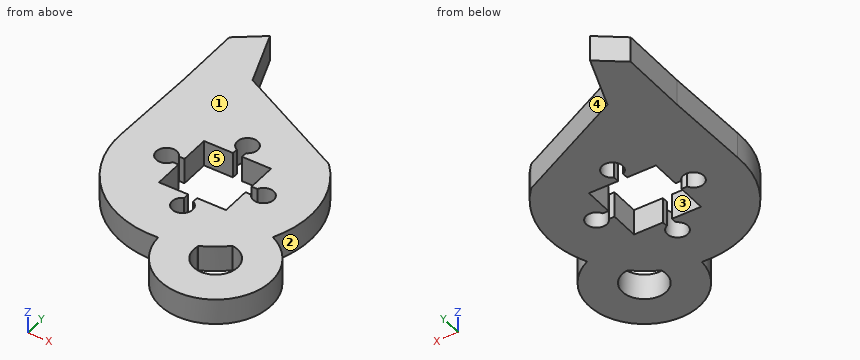
from build123d import *

# Parameters (mm, degrees)
BOSS_EXTRUDE1_DEPTH = 6.35
BOSS_EXTRUDE3_DEPTH = 6.35


with BuildPart() as part:
    # Sketch1 → Boss-Extrude1 (new body)
    with BuildSketch(Plane.XY):
        with BuildLine():
            Line((-23.080739782, 22.623363343), (-23.587362778, 1.111628824))
            ThreePointArc((-23.587362778, 1.111628824), (8.159769108, -22.158916254), (17.23339163, 16.143407769))
            Line((17.23339163, 16.143407769), (-11.238980923, 30.520917168))
            Line((-11.238980923, 30.520917168), (-16.457039411, 44.691234922))
            Line((-16.457039411, 44.691234922), (-23.120633834, 39.693776399))
            Line((-23.120633834, 39.693776399), (-23.080739782, 22.623363343))
        make_face()
        with BuildLine():
            ThreePointArc((1.1176, 9.657085657), (0, 14.478), (-1.1176, 9.657085657))
            Line((-1.1176, 9.657085657), (-1.1176, 8.255))
            Line((-1.1176, 8.255), (-8.255, 8.255))
            Line((-8.255, 8.255), (-8.255, 1.1176))
            Line((-8.255, 1.1176), (-9.657085657, 1.1176))
            ThreePointArc((-9.657085657, 1.1176), (-14.478, 0), (-9.657085657, -1.1176))
            Line((-9.657085657, -1.1176), (-8.255, -1.1176))
            Line((-8.255, -1.1176), (-8.255, -8.255))
            Line((-8.255, -8.255), (-1.1176, -8.255))
            Line((-1.1176, -8.255), (-1.1176, -9.657085657))
            ThreePointArc((-1.1176, -9.657085657), (0, -14.478), (1.1176, -9.657085657))
            Line((1.1176, -9.657085657), (1.1176, -8.255))
            Line((1.1176, -8.255), (8.255, -8.255))
            Line((8.255, -8.255), (8.255, -1.1176))
            Line((8.255, -1.1176), (9.657085657, -1.1176))
            ThreePointArc((9.657085657, -1.1176), (14.478, 0), (9.657085657, 1.1176))
            Line((9.657085657, 1.1176), (8.255, 1.1176))
            Line((8.255, 1.1176), (8.255, 8.255))
            Line((8.255, 8.255), (1.1176, 8.255))
            Line((1.1176, 8.255), (1.1176, 9.657085657))
        make_face(mode=Mode.SUBTRACT)
    extrude(amount=BOSS_EXTRUDE1_DEPTH)

    # Sketch2 → Boss-Extrude3 (add)
    with BuildSketch(Plane(origin=(0, 0, 0), x_dir=(-1, 0, 0), z_dir=(0, 0, -1))):
        with BuildLine():
            ThreePointArc((-13.902877587, -9.175702687), (-24.867617177, -32.651605631), (-1.941453441, -20.57954907))
            ThreePointArc((-1.941453441, -20.57954907), (-6.682478708, -17.156714595), (-10.105313182, -21.897739863))
            ThreePointArc((-10.105313182, -21.897739863), (-19.161295375, -26.666279881), (-14.830152685, -17.393147165))
            ThreePointArc((-14.830152685, -17.393147165), (-10.257792897, -13.748062475), (-13.902877587, -9.175702687))
        make_face()
    extrude(amount=-BOSS_EXTRUDE3_DEPTH)


solid = part.part
The model under review builds one solid part; all positions refer to its coordinate system, in mm. Face numbers are marked on the shaded views. A direction names the side the tool comes from. Coordinates: 2 decimals unless noted, no trailing zeros. Loops run counter-clockwise (first coordinate to the right, second up) from the corner with the lowest first, then second, coordinate; pieces in that order, holes last. Notation, with made-up numbers: M 39,20 L 80,20 A15 cw 80,34 Z; hole C 33.25,53 d4. An arc over 180 degrees is marked long. Put each result on its own line as item: value. Start each with the question number.
Q1. Add section B-B (x = 13). Write out the cut boundary in (y, z).
Q2. The part is to be moulded in two halves that separate along X. For the marked faces 1, 2 and 3, say which applies: +X half, -X half, draft (parallel to the pull), parting line (faces both ways), or undercut.
Q3. Clearance check with flat-ended pins moving along their axes: pin 1 (1.5 mm diameter, centred on y = -9, z = 2, fed in from +X); pin 2 (1.5 mm diameter, centred on x = -9, z = 2.5, fed in from +Y); pin 3 (1.5 mm diameter, centred on y = 29.5, z = 1, fed in from -X); pin 4 (4 mm diameter, centred on x = -1, y = 17.5, fed in from -Z). State where each tip first meets the part, or that it passes through.
Q4. Add section A-A (y = 0). Write out the cut boundary in (x, z), and give its area (3 significant figures).
Q5. Wall thickness on line 1 (X direction, y = 2, z = 4.5) (3 decimals); line 2 (Y direction, x = 1.5, z = 4) (3 decimals); line 3 (Y direction, x = -7, z = 5.5) (3 decimals): over which ranges is each line inside the solid? List them lowest first.
Q6. For the marked faces 4 and 5, list the 3-axis set-ups (+Z, -Z, +X, -X, +Y, -Y) from which the entire face can be reached by the end or side of a thin tool; tool diameter is ignored.
Q7. Add section D-D (z = 2.5). Count the separate pieces of the cut face and the enclosed holes in it, and give its area (3 significant figures).
Q8. Add section C-C (x = 0). Write out the cut boundary in (y, z), and give its area (3 significant figures).
Answers:
1. outline: M -36.21,0 L -27.58,0 L -27.58,6.35 L -36.21,6.35 Z; M -19.71,0 L -2.31,0 L -2.31,6.35 L -19.71,6.35 Z; M 2.31,0 L 18.28,0 L 18.28,6.35 L 2.31,6.35 Z
2. face 1: draft
2. face 2: +X half
2. face 3: undercut
3. pin 1: stops at x = 22.13
3. pin 2: stops at y = 29.77
3. pin 3: stops at x = -23.1
3. pin 4: stops at z = 0
4. outline: M -23.61,0 L -14.48,0 L -14.48,6.35 L -23.61,6.35 Z; M 14.48,0 L 23.61,0 L 23.61,6.35 L 14.48,6.35 Z
4. area: 116 mm^2
5. line 1: x = -23.566 to -13.504, -10.372 to -8.255, 8.255 to 10.372, 13.504 to 23.529
5. line 2: y = -23.566 to -13.988, -9.888 to -8.255, 8.255 to 9.888, 13.988 to 24.088
5. line 3: y = -22.552 to -8.255, 8.255 to 28.38
6. face 4: +Z, -Z, +X, +Y
6. face 5: +Z, -Z
7. separate pieces: 1
7. enclosed holes: 2
7. area: 2,070 mm^2
8. outline: M -23.61,0 L -14.48,0 L -14.48,6.35 L -23.61,6.35 Z; M 14.48,0 L 24.85,0 L 24.85,6.35 L 14.48,6.35 Z
8. area: 124 mm^2
